The listing builds one solid part. Answer for the finished solid, in the listing's coordinates (mm). Face numbers are marked on the shaded views. A direction names the side the tool comes from. Round coordinates to 2 decimals unless told otherwise and drop trailing zeros. Order: outer loops, then holes, each group sorted by start corner. A loop starts at its lowest first (then second) coordinate and runs counter-clockwise, first axis right, second up. Notation, with made-up numbers: (-8.75, -10.5) - (12.25, -10.5) arc R9 ccw to (12.25, -6.5) - close; hole circle Ø4 at (-27, 10.5). An arc over 180 degrees is marked (long way). Use CSV: the item, a comma, the result in double quotes. Start each with the question number.
Item 1: Find section A-A, the plane x = -5.9. Give the vertices of the cut face in (y, z).
Item 2: Flat-ended cylindrical pins translate along their axes: P1, Ø2, axis at x = -5.9, z = 0, coming from the +Y side; P2, Ø1.5, axis at y = 3, z = 7.5, coming from the -X side. Find the tip coordinate at first contact, or state that the pin passes through.
Item 3: Find section C-C, the plane y = 4.35. Give the vertices of the cut face in (x, z).
Item 4: Find section D-D, the plane x = -15. Give the vertices of the cut face in (y, z).
Item 5: Determine the mould class of the marked faces 1, 2 and 3 for opening direction X: +X half, -X half, draft (parallel to the pull), parting line (faces both ways), or undercut.
Item 6: Find section B-B, the plane z = -2.5. Give the vertices of the cut face in (x, y).
Item 7: Straight lines are drawn through the part: line 1 along X through (y, z) = (2.25, 0); line 2 along X through (y, z) = (2.1, -5.5); line 3 along Z through (x, y) = (-2, 0.3). For each, find the intervals that lie inside material, in ascending order. Write a range as [from, to].
Item 8: For the marked faces 4 and 5, determine the directions among +Z, -Z, +X, -X, +Y, -Y from which every point of the face is accessible in a straight line to the end or side of a thin tool.
```python
from build123d import *

# Parameters (mm, degrees)
SKETCH1_W           = 55
SKETCH1_H           = 22
BOSS_EXTRUDE1_DEPTH = 5
SKETCH2_R           = 2.5
CUT_EXTRUDE1_DEPTH  = 5
FILLET1_R           = 5
SKETCH4_R           = 1.1
SKETCH4_W           = 24
SKETCH4_H           = 14
CUT_EXTRUDE2_DEPTH  = 5


with BuildPart() as part:
    # Sketch1 → Boss-Extrude1 (new body)
    with BuildSketch(Plane(origin=(0, 0, 0), x_dir=(1, 0, 0), z_dir=(0, 1, 0))):
        with Locations((-2.5, 0)):
            Rectangle(SKETCH1_W, SKETCH1_H)
    extrude(amount=BOSS_EXTRUDE1_DEPTH)

    # Sketch2 → Cut-Extrude1 (cut)
    with BuildSketch(Plane(origin=(0, 5, 0), x_dir=(1, 0, 0), z_dir=(0, 1, 0))):
        with Locations(Location((-25, 5.5, 0), (0, 0, 270))):
            Circle(SKETCH2_R)
        with Locations(Location((-15, 5.5, 0), (0, 0, 270))):
            Circle(SKETCH2_R)
        with Locations(Location((-25, -5.5, 0), (0, 0, 270))):
            Circle(SKETCH2_R)
        with Locations(Location((-15, -5.5, 0), (0, 0, 270))):
            Circle(SKETCH2_R)
    extrude(amount=-CUT_EXTRUDE1_DEPTH, mode=Mode.SUBTRACT)

    # Fillet1
    fillet1_edges = [part.edges().sort_by_distance(p)[0] for p in [
        (-30, 2.5, -11),
        (25, 2.5, -11),
        (25, 2.5, 11),
        (-30, 2.5, 11),
    ]]
    fillet(fillet1_edges, radius=FILLET1_R)

    # Sketch4 → Cut-Extrude2 (cut)
    with BuildSketch(Plane(origin=(0, 5, 0), x_dir=(1, 0, 0), z_dir=(0, 1, 0))):
        with Locations(Location((21.9, 0, 0), (0, 0, 270))):
            Circle(SKETCH4_R)
        with Locations(Location((-5.9, 0, 0), (0, 0, 90))):
            Circle(SKETCH4_R)
        with Locations((8, 0)):
            Rectangle(SKETCH4_W, SKETCH4_H)
    extrude(amount=-CUT_EXTRUDE2_DEPTH, mode=Mode.SUBTRACT)


solid = part.part
```
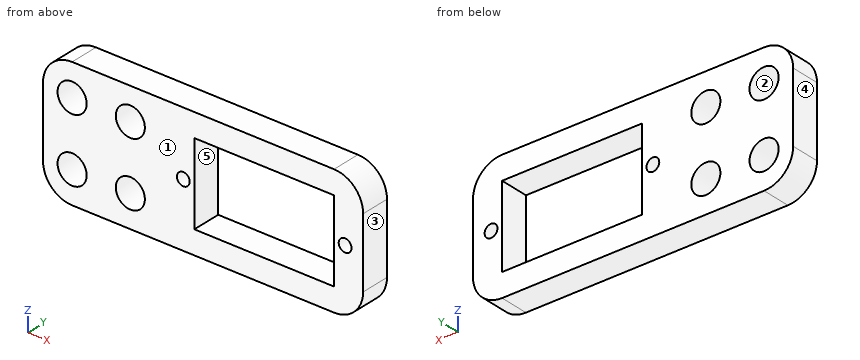
Worked out:
1,outline,"(0, -11) - (5, -11) - (5, -1.1) - (0, -1.1) - close; (0, 1.1) - (5, 1.1) - (5, 11) - (0, 11) - close"
2,P1,"passes through"
2,P2,"stops at x = -29.94"
3,outline,"(-30, -6) arc R5 ccw to (-25, -11) - (20, -11) arc R5 ccw to (25, -6) - (25, 6) arc R5 ccw to (20, 11) - (-25, 11) arc R5 ccw to (-30, 6) - close; hole circle Ø5 at (-25, -5.5); hole circle Ø5 at (-25, 5.5); hole circle Ø5 at (-15, -5.5); hole circle Ø5 at (-15, 5.5); hole circle Ø2.2 at (-5.9, 0); hole (-4, -7) - (20, -7) - (20, 7) - (-4, 7) - close; hole circle Ø2.2 at (21.9, 0)"
4,outline,"(0, -11) - (5, -11) - (5, -8) - (0, -8) - close; (0, -3) - (5, -3) - (5, 3) - (0, 3) - close; (0, 8) - (5, 8) - (5, 11) - (0, 11) - close"
5,face 1,"draft"
5,face 2,"undercut"
5,face 3,"+X half"
6,outline,"(-30, 0) - (-4, 0) - (-4, 5) - (-30, 5) - close; (20, 0) - (25, 0) - (25, 5) - (20, 5) - close"
7,line 1,"x = [-30, -7], [-4.8, -4], [20, 20.8], [23, 25]"
7,line 2,"x = [-30, -27.5], [-22.5, -17.5], [-12.5, -4], [20, 25]"
7,line 3,"z = [-11, -7], [7, 11]"
8,face 4,"+Z, -Z, -X, +Y, -Y"
8,face 5,"+Y, -Y"
